Drawing for the job (mm, zero at the part's lowest x, y, z). Coordinates: 2 decimals unless noted, no trailing zeros. Write each loop counter-clockwise with the first axis right and the second up, starting at its lowest first coordinate (ties: lowest second). Pieces come first, ordered by that corner, then holes. Notation, with made-up numbers: (5.25, 60) - (29.25, 60) arc R27 ccw to (29.25, 85) - close; hole circle Ø1 at (-35, -39). An arc over 180 degrees is marked (long way). Write each question's results on one line, items separated by ' | '.
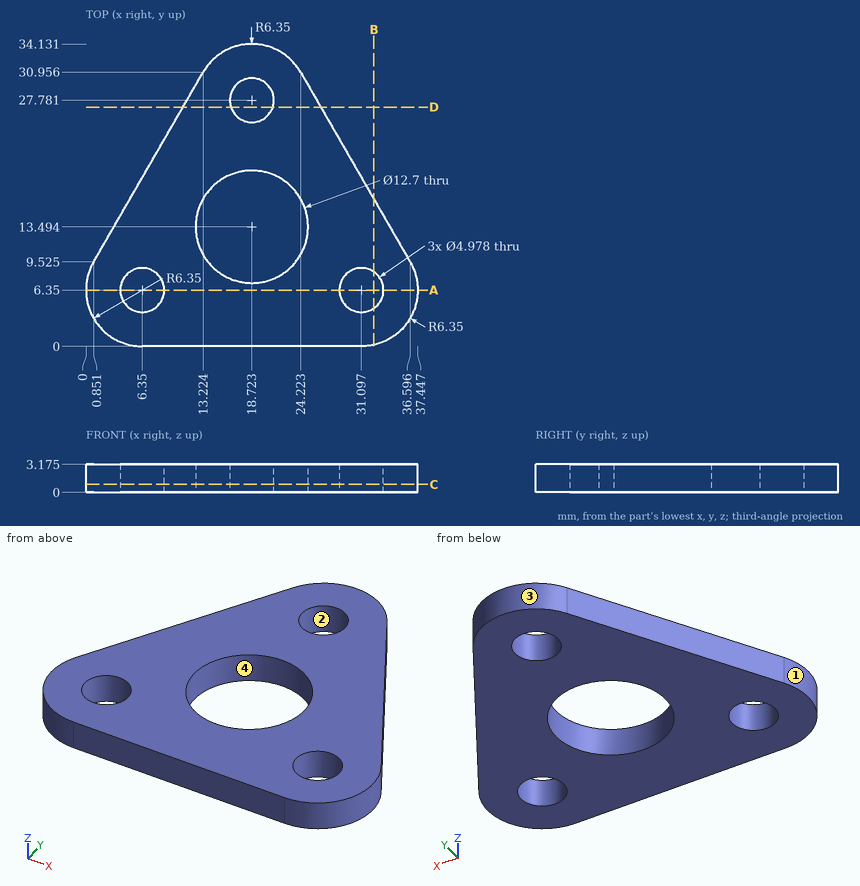
(1) Two-plate mould, pull along X, no slides. Class the marked faces 1, 2, 3 and 4: released by +X, released by -X, zero draft, split by the parting line, or undercut.
Return value:
face 1: released by -X | face 2: undercut | face 3: split by the parting line | face 4: undercut
(2) Wall check: line 1 (X direction, y = 18.5, z = 2.45) (1 decimal); line 2 (Y direction, x = 13.5, z = 0.75) (1 decimal); line 3 (Y direction, x = 15.5, z = 3) (1 decimal). Give the ranges that are in metal, low to high. Write a range as from..to.
Return value:
line 1: x = 6..14.8, 22.6..31.4 | line 2: y = 0..9.9, 17.1..31.4 | line 3: y = 0..8, 19..33.3
(3) Saw through at D-D on y = 27. Write the cut outline in (x, z) (1 decimal), then the cut area to 3 significant figures.
Return value:
outline: (10.9, 0) - (16.4, 0) - (16.4, 3.2) - (10.9, 3.2) - close; (21.1, 0) - (26.5, 0) - (26.5, 3.2) - (21.1, 3.2) - close | area: 34.4 mm^2
(4) Saw through at C-C on z = 0.9. Count the separate pieces of the cut face and the enclosed holes in it, then the cut area to 3 significant figures.
Return value:
separate pieces: 1 | enclosed holes: 4 | area: 678 mm^2
(5) Flat gauge pins, fed straight in: P1, Ø5, axis at x = 30, y = 29, coming from the +Z side; P2, Ø6.5, axis at x = 31.1, y = 6.35, coming from the +Z side (3 decimals). Where does each tip first touch, or does it go through?
Return value:
P1: passes through | P2: stops at z = 3.175
(6) Saw through at A-A on y = 6.35. Write the cut outline in (x, z) (1 decimal).
Return value:
outline: (0, 0) - (3.9, 0) - (3.9, 3.2) - (0, 3.2) - close; (8.8, 0) - (28.6, 0) - (28.6, 3.2) - (8.8, 3.2) - close; (33.6, 0) - (37.4, 0) - (37.4, 3.2) - (33.6, 3.2) - close
(7) Saw through at B-B on x = 32.5. Write the cut outline in (y, z) (1 decimal), then the cut area to 3 significant figures.
Return value:
outline: (0.2, 0) - (4.3, 0) - (4.3, 3.2) - (0.2, 3.2) - close; (8.4, 0) - (16.6, 0) - (16.6, 3.2) - (8.4, 3.2) - close | area: 39.2 mm^2
